Read the model definition and answer for the solid it produces. Units are mm, in the model's axes. A direction names the side the tool comes from. Round coordinates to 2 decimals unless told otherwise and drop trailing zeros. Write each loop counter-clockwise with the first axis right and the second up, starting at its lowest first coordinate (ties: lowest second). Pieces come first, ordered by that corner, then holes. Notation, with made-up numbers: (-21, 75.5) - (-12, 75.5) arc R19 ccw to (-12, 82.5) - close; hole circle Ø7 at (65, 47.5). An arc over 180 degrees is marked (long way). One line per item, written item: value. Start each with the question number.
(1) The mould has two halves that part along X. Classify faces 5 (the face through (11.355, -12.799, 11.198)), 6 (the face through (0.12, 10.6, 5.57)), 7 (the face through (18.5, 25.2, 2.5)), 8 (the face through (22.675, 0, 2)): +X half, -X half, draft (parallel to the pull), parting line (faces both ways), or undercut.
(2) For faces 1 (the face through (-9.725, 8.028, 14.626)), 2 (the face through (6.766, -13.29, 9.93)), 3 (the face through (-22.105, 33.074, 2.535)), 4 (the face through (9.725, 8.028, 14.626)), determine the directions among +Z, -Z, +X, -X, +Y, -Y from which every point of the face is accessible in a straight line to the end or side of a thin tool.
(3) Flat-ended cylindrical pins translate along their axes: pin 1 Ø4 at (x, z) = (2, 9.5) entering from -Y; pin 2 Ø8 at (x, z) = (-14, 11) entering from +Y; pin 3 Ø10 at (x, y) = (17, 28) entering from +Z; pin 4 Ø5 at (x, y) = (-17, -28) entering from +Z. Find the tip coordinate at first contact, or state that the pin passes through.
(4) A cutting plane is placed at C-C, the plane y = 28. Determine the outline of the cut face in (x, z) (3 decimals).
(5) A cutting plane is placed at B-B, the plane x = 17. Determine the outline of the cut face in (y, z) (3 decimals), plus the area to 3 significant figures.
(6) A cutting plane is placed at A-A, the plane z = 11.25. State how many separate pieces and enclosed holes the cut face has, plus the area to 3 significant figures.
(7) Find the intervals of material crossed by L1, parallel to Y at x = -7.56, z = 8.25; L2, parallel to Y at x = 17, z = 3.9 (3 decimals); L3, parallel to Z at x = -19.5, y = 16, in increasing order.
(8) A cutting plane is placed at D-D, the plane z = 1.5. Determine the outline of the cut face in (x, y) (3 decimals).
from build123d import *

# Parameters (mm, degrees)
SKETCH1_W           = 45.35
SKETCH1_H           = 67.35
SKETCH1_R           = 3.175
BOSS_EXTRUDE1_DEPTH = 5
SKETCH2_R           = 4
SKETCH2_R_2         = 1.05
SKETCH2_W           = 21.12
SKETCH2_H           = 4
BOSS_EXTRUDE2_DEPTH = 10
FILLET1_R           = 2
FILLET2_R           = 2
FILLET3_R           = 2.5


with BuildPart() as part:
    # Sketch1 → Boss-Extrude1 (new body)
    with BuildSketch(Plane.XY):
        Rectangle(SKETCH1_W, SKETCH1_H)
        with Locations((-17, 28)):
            Circle(SKETCH1_R, mode=Mode.SUBTRACT)
        with Locations((17, 28)):
            Circle(SKETCH1_R, mode=Mode.SUBTRACT)
        with Locations((17, -28)):
            Circle(SKETCH1_R, mode=Mode.SUBTRACT)
        with Locations((-17, -28)):
            Circle(SKETCH1_R, mode=Mode.SUBTRACT)
    extrude(amount=BOSS_EXTRUDE1_DEPTH)

    # Sketch2 → Boss-Extrude2 (add)
    # profile 1 of 3: a face of its own
    with BuildSketch(Plane.XY.offset(5)):
        with Locations((7.54, -14)):
            Circle(SKETCH2_R)
        with Locations((7.54, -14)):
            Circle(SKETCH2_R_2, mode=Mode.SUBTRACT)
    # profile 2 of 3: a face of its own
    with BuildSketch(Plane.XY.offset(5)):
        with Locations((-7.56, -14)):
            Circle(SKETCH2_R)
        with Locations((-7.56, -14)):
            Circle(SKETCH2_R_2, mode=Mode.SUBTRACT)
    # profile 3 of 3: a face of its own
    with BuildSketch(Plane.XY.offset(5)):
        with Locations((0, 8)):
            Rectangle(SKETCH2_W, SKETCH2_H)
    extrude(amount=BOSS_EXTRUDE2_DEPTH)

    # Fillet1
    fillet1_edges = [part.edges().sort_by_distance(p)[0] for p in [
        (22.675, -33.675, 2.5),
        (-22.675, -33.675, 2.5),
        (-22.675, 33.675, 2.5),
        (22.675, 33.675, 2.5),
    ]]
    fillet(fillet1_edges, radius=FILLET1_R)

    # Fillet2
    fillet2_edges = [part.edges().sort_by_distance(p)[0] for p in [
        (0, 6, 5),
        (-10.56, 6, 10),
        (10.56, 8, 5),
        (10.56, 6, 10),
        (10.56, 10, 10),
        (-10.56, 8, 15),
        (-10.56, 10, 10),
        (10.56, 8, 15),
        (-10.56, 8, 5),
        (0, 10, 5),
    ]]
    fillet(fillet2_edges, radius=FILLET2_R - 0.0001)  # a hair under: the kernel refuses the full size

    # Fillet3
    fillet3_edges = [part.edges().sort_by_distance(p)[0] for p in [
        (3.54, -14, 5),
        (-11.56, -14, 5),
    ]]
    fillet(fillet3_edges, radius=FILLET3_R)


solid = part.part
Here are the results:
1. face 5: undercut
1. face 6: draft
1. face 7: undercut
1. face 8: +X half
2. face 1: +Z, -X, +Y
2. face 2: +Z
2. face 3: +Z, -Z, -X, +Y
2. face 4: +Z, +X, +Y
3. pin 1: y = -15.86
3. pin 2: y = 9.39
3. pin 3: z = 5
3. pin 4: through
4. outline: (-22.675, 0) - (-20.175, 0) - (-20.175, 5) - (-22.675, 5) - close; (-13.825, 0) - (13.825, 0) - (13.825, 5) - (-13.825, 5) - close; (20.175, 0) - (22.675, 0) - (22.675, 5) - (20.175, 5) - close
5. outline: (-33.675, 0) - (-31.175, 0) - (-31.175, 5) - (-33.675, 5) - close; (-24.825, 0) - (24.825, 0) - (24.825, 5) - (-24.825, 5) - close; (31.175, 0) - (33.675, 0) - (33.675, 5) - (31.175, 5) - close
5. area: 273 mm²
6. separate pieces: 3
6. enclosed holes: 2
6. area: 175 mm²
7. L1: -18 to -15.05, -12.95 to -10, 6 to 10
7. L2: -33.675 to -31.175, -24.825 to 24.825, 31.175 to 33.675
7. L3: 0 to 5
8. outline: (-22.675, -31.675) arc R2 ccw to (-20.675, -33.675) - (20.675, -33.675) arc R2 ccw to (22.675, -31.675) - (22.675, 31.675) arc R2 ccw to (20.675, 33.675) - (-20.675, 33.675) arc R2 ccw to (-22.675, 31.675) - close; hole circle Ø6.35 at (-17, -28); hole circle Ø6.35 at (-17, 28); hole circle Ø6.35 at (17, -28); hole circle Ø6.35 at (17, 28)
